Source: CAD feature listing. Evaluate the final solid. Frame: model axes, mm. Face numbers are marked on the shaded views. A direction names the side the tool comes from. Give positions to 0.01 mm unless a question says otherwise; leave off trailing zeros. Loops run counter-clockwise (first coordinate to the right, second up) from the corner with the lowest first, then second, coordinate; pieces in that order, holes last. Notation, with made-up numbers: (80, 7) -> (109, 7) arc R11 ccw to (109, 17) -> close; hole circle Ø9 at (-36.5, 65). An arc over 180 degrees is marked (long way). Return JSON: item names as keys, results as strings. Group by question number.
(1) Cut plane A-A on z = 0.5. Return loops of the section in (x, y).
(2) Cut plane C-C on x = 4. Return loops of the section in (y, z).
(3) Pin query (flat end, axial travel): pin 1 (3 mm diameter, centred on x = 23, z = 4.5, fed in from -Y); pin 2 (4 mm diameter, centred on x = 22.5, y = 7, fed in from +Z). Return the tip coordinate at first contact, or that it passes through.
(4) Cut plane B-B on y = 6.75. Return loops of the section in (x, z).
(5) Access query for the marked faces 1 and 2. Directions: +Z, -Z, +X, -X, +Y, -Y. A direction counts if a zero-diameter tool reaches every point of the face in a straight line with its end or side. Return the directions, or none.
(6) Ray query, line 1 (X direction, y = 7.5, z = 3); line 2 (Z direction, x = 2, y = 2); line 3 (X direction, y = 9.75, z = -4.25). Return the intervals inside material, ascending. Write a range as from..to.
```python
from build123d import *

# Parameters (mm, degrees)
BOSS_EXTRUDE1_DEPTH = 10
FILLET1_R           = 2


with BuildPart() as part:
    # Sketch1 → Boss-Extrude1 (new body)
    with BuildSketch(Plane(origin=(0, 0, 0), x_dir=(1, 0, 0), z_dir=(0, 1, 0))):
        Polygon((0, 0), (8, 0), (8, -6), (19.75, -6), (19.75, 0), (27.75, 0), (27.75, -6), (32.75, -6), (32.75, 6), (-5, 6), (-5, -6), (0, -6), align=None)
    extrude(amount=BOSS_EXTRUDE1_DEPTH)

    # Fillet1
    fillet1_edges = [part.edges().sort_by_distance(p)[0] for p in [
        (-5, 5, -6),
        (32.75, 5, -6),
    ]]
    fillet(fillet1_edges, radius=FILLET1_R)


solid = part.part
```
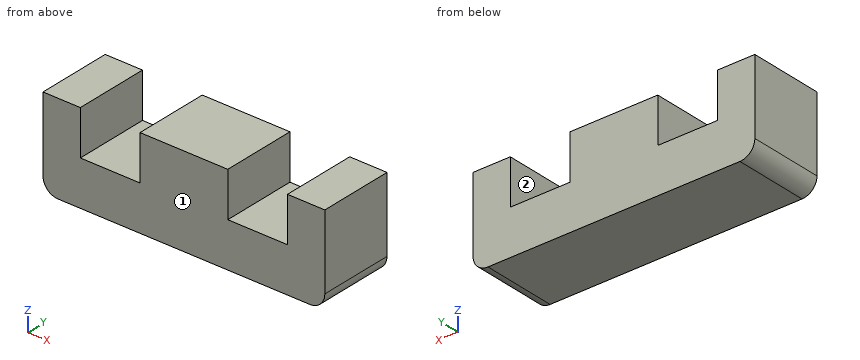
Answers:
{
 "1": {"outline": "(-5, 0) -> (0, 0) -> (0, 10) -> (-5, 10) -> close; (8, 0) -> (19.75, 0) -> (19.75, 10) -> (8, 10) -> close; (27.75, 0) -> (32.75, 0) -> (32.75, 10) -> (27.75, 10) -> close"},
 "2": {"outline": "(0, -6) -> (10, -6) -> (10, 0) -> (0, 0) -> close"},
 "3": {"pin 1": "through", "pin 2": "z = 0"},
 "4": {"outline": "(-5, -4) arc R2 ccw to (-3, -6) -> (30.75, -6) arc R2 ccw to (32.75, -4) -> (32.75, 6) -> (27.75, 6) -> (27.75, 0) -> (19.75, 0) -> (19.75, 6) -> (8, 6) -> (8, 0) -> (0, 0) -> (0, 6) -> (-5, 6) -> close"},
 "5": {"face 1": "+Z, -Z, +X, -X, -Y", "face 2": "+Z, +Y, -Y"},
 "6": {"line 1": "-5..0, 8..19.75, 27.75..32.75", "line 2": "-6..0", "line 3": "-4.98..32.73"}
}
